Autodesk Inventor part; units mm, degrees
ref_plane "YZ Plane" through (0, 0, 0) normal (1, 0, 0) x (0, 1, 0)
ref_plane "XZ Plane" through (0, 0, 0) normal (0, 1, 0) x (-1, 0, 0)
ref_plane "XY Plane" through (0, 0, 0) normal (0, 0, 1) x (1, 0, 0)
ref_plane "Work Plane4" through (23.7495, -12.4998, 8) normal (0, 0, -1) x (0.866, 0.5, 0)
sketch "Sketch9" plane through (23.7495, -12.4998, 8) normal (0, 0, -1) x (0.866, 0.5, 0)
  circle A0 centre (-36.9735, 7.7008) radius 1.3002
  circle A1 centre (8.3375, 7.7008) radius 1.3002
  circle A2 centre (23.3378, -18.28) radius 1.3
  circle A3 centre (-14.318, -22.6998) radius 21.9102
  circle A4 centre (-51.9737, -18.28) radius 1.3001
  line L0 (-27.63, -57.387) -> (-29.04, -59.377)
  circle A5 centre (-29.3181, -57.5206) radius 1.3001
  circle A6 centre (0.6822, -57.5205) radius 1.3
  circle A7 centre (11.5075, -7.7902) radius 1.3002
  line L1 (-33.586, -63.403) -> (4.877, -63.403) construction
  line L2 (-39.9342, 14.3381) -> (-59.166, -18.972) construction
  line L3 (30.566, -19.035) -> (11.3349, 14.275) construction
  line L4 (-14.3189, -92.6998) -> (-74.9393, 12.301) construction
  line L5 (-74.9393, 12.301) -> (46.3042, 12.2995) construction
  line L6 (46.3042, 12.2995) -> (-14.3189, -92.6998) construction
  line L7 (41.198, -34.545) -> (23.698, -64.855) construction
  line L8 (2.5961, -63.403) -> (-31.2329, -63.403)
  line L9 (-31.2329, -63.403) -> (-58.0252, -16.9961)
  line L10 (-58.0252, -16.9961) -> (-41.1106, 12.3006)
  line L11 (-41.1106, 12.3006) -> (12.4752, 12.2999)
  line L12 (12.4752, 12.2999) -> (29.3894, -16.997)
  line L13 (29.3894, -16.997) -> (2.5961, -63.403)
  point P0 (-14.318, -22.6998)
  dimension "d56" = 35
extrude "Extrusion4" add sketch "Sketch9" along normal blind 3
sketch "Sketch10" plane through (23.7495, -12.4998, 5) normal (0, 0, -1) x (-0.866, -0.5, 0)
  circle A0 centre (14.318, 22.6998) radius 21.9102
  circle A1 centre (36.9735, -7.7008) radius 1.3002
  circle A2 centre (-8.3375, -7.7008) radius 1.3002
  circle A3 centre (-11.5075, 7.7902) radius 1.3002
  circle A4 centre (29.3181, 57.5206) radius 1.3001
  circle A5 centre (51.9737, 18.28) radius 1.3001
  circle A6 centre (-23.3378, 18.28) radius 1.3
  circle A7 centre (-0.6822, 57.5205) radius 1.3
  line L0 (31.2329, 63.403) -> (-2.5961, 63.403)
  line L1 (-2.5961, 63.403) -> (-29.3894, 16.997)
  line L2 (-29.3894, 16.997) -> (-12.4752, -12.2999)
  line L3 (-12.4752, -12.2999) -> (41.1106, -12.3006)
  line L4 (41.1106, -12.3006) -> (58.0252, 16.9961)
  line L5 (58.0252, 16.9961) -> (31.2329, 63.403)
  line L6 (32.318, -14.6138) -> (-3.682, -14.6138)
  line L7 (-3.682, -14.6138) -> (-3.682, -4.5139)
  line L8 (-3.682, -4.5139) -> (32.318, -4.5139)
  line L9 (32.318, -4.5139) -> (32.318, -14.6138)
  point P0 (14.318, 22.6998)
  dimension "d59" = 18
  dimension "d60" = 18
extrude "Extrusion5" cut sketch "Sketch10" against normal through all contours L9 L6 L7 L3 | L3 L7 L8 L9
pattern_circular "Circular Pattern1" count 3 over 360 about axis through (0, 0, 8) along (0, 0, -1) of "Extrusion5"
sketch "Sketch11" plane through (23.7495, -12.4998, 5) normal (0, 0, -1) x (-0.866, -0.5, 0)
  line L0 (23.469, 56.8503) -> (-7.8173, 38.7876)
  line L1 (-15.8275, 24.9136) -> (5.167, -11.4508)
  line L2 (5.167, -11.4508) -> (48.4685, 13.5488)
  line L3 (48.4685, 13.5488) -> (23.469, 56.8503)
  line L4 (23.469, 56.8503) -> (5.167, -11.4508) construction
  line L5 (-19.8325, 31.8507) -> (48.4685, 13.5488) construction
  line L6 (-2.59, 41.8055) -> (-7.8173, 38.7876)
  circle A0 centre (14.318, 22.6998) radius 21.9102
  line L7 (-0.2497, 51.8951) -> (-18.2497, 20.7181)
  line L8 (-3.682, -4.5139) -> (32.318, -4.5139)
  point P0 (14.318, 22.6998)
  point P1 (1.1621, -4.5139)
  point P2 (17.1824, -4.5139)
  dimension "d66" = 50
  dimension "d67" = 50
extrude "Extrusion6" add sketch "Sketch11" along normal blind 3 contours L3 L2 L8 L1 L7 L0
sketch "Sketch12" plane through (23.7495, -12.4998, 2) normal (0, 0, -1) x (-0.866, -0.5, 0)
  circle A0 centre (37.2753, 11.9362) radius 2.65
  circle A1 centre (39.5813, 20.5422) radius 2.65
  circle A2 centre (25.0816, 45.657) radius 2.65
  circle A3 centre (16.4756, 47.9631) radius 2.65
  circle A4 centre (-10.9453, 24.8574) radius 2.65
  circle A5 centre (3.5544, -0.2575) radius 2.65
  circle A6 centre (12.1604, -2.5635) radius 2.65
  circle A7 centre (-8.6393, 33.4633) radius 2.65
  point P0 (14.318, 22.6998)
hole "Hole4" at (-20.8, -14.5, 2) at (-14.5, -20.8, 2) at (20.8, -14.5, 2) at (20.8, 14.5, 2) at (-14.5, 20.8, 2) at (-20.8, 14.5, 2) direction (0, 0, 1) diameter 4.8 end through all
properties part number "20_Cube_Insert_Openflexure_Deltastage_Adapter"
Model file for the job. Use its own axes, mm. A direction names the side the tool comes from. Coordinates: 2 decimals unless noted, no trailing zeros. Loops run counter-clockwise (first coordinate to the right, second up) from the corner with the lowest first, then second, coordinate; pieces in that order, holes last. Notation, with made-up numbers: (77.25, 66.25) -> (99.25, 66.25) arc R24 cw to (99.25, 102.25) -> close; hole circle Ø7 at (38.25, 53.25). An arc over 180 degrees is marked (long way). Answer as a JSON object with one key per item and string values.
Q1. Cut at B-B (y = 3). List the corners of the cut face in (x, z).
Report:
{"outline": "(-27.21, 5) -> (-25, 5) -> (-25, 2) -> (-21.7, 2) -> (-21.7, 8) -> (-27.21, 8) -> close; (21.7, 2) -> (25, 2) -> (25, 5) -> (40.7, 5) -> (40.7, 8) -> (21.7, 8) -> close"}
Q2. Cut at A-A (x = -14.5). List the corners of the cut face in (y, z), and give its area (3 significant figures).
Report:
{"outline": "(-38.63, 5) -> (-25, 5) -> (-25, 2) -> (-23.2, 2) -> (-23.2, 8) -> (-38.63, 8) -> close; (-18.4, 2) -> (-16.43, 2) -> (-16.43, 8) -> (-18.4, 8) -> close; (16.43, 2) -> (18.4, 2) -> (18.4, 8) -> (16.43, 8) -> close; (23.2, 2) -> (25, 2) -> (25, 5) -> (38.63, 5) -> (38.63, 8) -> (23.2, 8) -> close", "area": "127 mm2"}
Q3. Flat gauge pins, fed straight in: P1, Ø3.5, axis at x = -30.4, y = -22.66, coming from the -Z side; P2, Ø3, axis at x = -14.5, y = 20.8, coming from the +Z side; P3, Ø3.5, axis at x = -13.5, z = 4, coming from the +Y side; P4, Ø2.5, axis at y = -8.5, z = 3.5, coming from the -X side. Where does each tip first touch, or does it go through?
Report:
{"P1": "stops at z = 5", "P2": "passes through", "P3": "stops at y = 40.03", "P4": "stops at x = -25"}
Q4. Cut at D-D (y = -7). List the corners of the cut face in (x, z).
Report:
{"outline": "(-27.21, 5) -> (-25, 5) -> (-25, 2) -> (-20.76, 2) -> (-20.76, 8) -> (-27.21, 8) -> close; (20.76, 2) -> (25, 2) -> (25, 5) -> (40.7, 5) -> (40.7, 8) -> (20.76, 8) -> close"}
Q5. Cut at C-C (z = 3.5). List the corners of the cut face in (x, y).
Report:
{"outline": "(-25, -25) -> (11.13, -25) -> (25, -16.99) -> (25, 16.99) -> (11.13, 25) -> (-25, 25) -> close; hole circle Ø4.8 at (-20.8, -14.5); hole circle Ø4.8 at (-20.8, 14.5); hole circle Ø43.82 at (0, 0); hole circle Ø4.8 at (-14.5, -20.8); hole circle Ø4.8 at (-14.5, 20.8); hole circle Ø4.8 at (20.8, -14.5); hole circle Ø4.8 at (20.8, 14.5)"}
Q6. Pull direction X, two halves, no side cores. Call faces 4 (the flat face through (-31, -18, 6)), 5 (the flat face through (31.115, 17.892, 6.479)), 6 (the flat face through (36.842, -19.143, 6.521)), 7 (the cylindrical face through (28.667, -0.6, 6.521)): released by +X, released by -X, zero draft, split by the parting line, or undercut.
Report:
{"face 4": "zero draft", "face 5": "undercut", "face 6": "released by +X", "face 7": "undercut"}
Q7. Probe probe 1 along X at (y, z) = (14.5, 6.2); probe 2 along Y at (x, z) = (-31.5, 5.4); probe 3 along X at (y, z) = (5, 5.75). List the from-to ranges inside material, lowest first.
Report:
{"probe 1": "x = -27.21 to -23.2, -18.4 to -16.43, 16.43 to 18.4, 23.2 to 33.62, 36.02 to 40.7", "probe 2": "y = -28.81 to -23.35, -21.96 to -18, 18 to 21.96, 23.35 to 28.81", "probe 3": "x = -27.21 to -21.33, 21.33 to 40.7"}
Q8. 3-axis set-ups, long thin cutter, end or side, ignore diameter. For faces 1 (the flat face through (27, -1, 5)), 2 (the flat face through (-27.214, 0, 6)), 3 (the cylindrical face through (36.11, -14.83, 6.52)): which of +Z, -Z, +X, -X, +Y, -Y reach the whole face in a straight line?
Report:
{"face 1": "-Z", "face 2": "+Z, -Z, -X", "face 3": "+Z, -Z"}
